```python
from build123d import *

# Parameters (mm, degrees)
F1_DEPTH = 3.175
F2_R     = 3.7719
F3_DEPTH = 1.27
F4_W     = 1.5875
F4_H     = 2.54
F5_DEPTH = 3.175


with BuildPart() as f1:
    # F0 (on Front) → F1 (new body)
    with BuildSketch(Plane.XZ):
        with BuildLine():
            ThreePointArc((39.878, 0), (0, 39.878), (-39.878, 0))
            Line((-39.878, 0), (-39.878, -14.986))
            Line((-39.878, -14.986), (39.878, -14.986))
            Line((39.878, -14.986), (39.878, 0))
        make_face()
    extrude(amount=F1_DEPTH)

    # F2 (on face) → F3 (cut)
    with BuildSketch(Plane.XZ.offset(3.175)):
        with Locations((-12.7, -7.493)):
            Circle(F2_R)
        with Locations((12.7, -7.493)):
            Circle(F2_R)
    extrude(amount=-F3_DEPTH, mode=Mode.SUBTRACT)

    # F4 (on face) → F5 (join)
    with BuildSketch(Plane.XZ.offset(3.175)):
        with Locations((-4.15925, -16.256)):
            Rectangle(F4_W, F4_H)
        with Locations((4.15925, -16.256)):
            Rectangle(F4_W, F4_H)
    extrude(amount=-F5_DEPTH)


solid = f1.part
```
Input: part model. Units: mm. Frame: model coordinates. A direction names the side the tool comes from. Coordinates: 2 decimals unless noted, no trailing zeros. Write each loop counter-clockwise with the first axis right and the second up, starting at its lowest first coordinate (ties: lowest second). Pieces come first, ordered by that corner, then holes.
1) Section B-B on x = -12.7. Output: boundary loops of the cut face in (y, z) (3 decimals), and give its area (3 significant figures).
2) Pin query (flat end, axial travel): pin 1 Ø7 at (x, z) = (12.7, -7.493) entering from +Y; pin 2 Ø2.5 at (x, z) = (12.5, -6.5) entering from -Y (3 decimals); pin 3 Ø0.8 at (y, z) = (-1.5, -16.5) entering from +X; pin 4 Ø0.8 at (y, z) = (-2, -16.5) entering from -X. Return the tip coordinate at first contact, or that it passes through.
3) Section A-A on y = -0.55. Output: boundary loops of the cut face in (x, z).
4) Section D-D on x = 0. Output: boundary loops of the cut face in (y, z) (3 decimals), and give its area (3 significant figures).
5) Mould query, pull axis X, two halves, no side actions, for faces 4 (the cylindrical face through (11.882, -2.549, -11.175)), 5 (the flat face through (4, -2, -17.526)), 6 (the cylindrical face through (0.88, -1.57, 39.87)), 7 (the flat face through (-13, -1.905, -7)). Classes: pulls with the +X half, pulls with the -X half, needs draft (parallel to the pull), parting line crosses it, or undercut.
6) Set-up query: faces 1 (the flat face through (-4.953, -2, -16)), 2 (the flat face through (4.953, -2, -16)), 3 (the flat face through (-3.366, -2, -16)). Return all of +Z, -Z, +X, -X, +Y, -Y with unobstructed straight access to the full face (end or side cutting, diameter ignored); none if empty.
7) Section C-C on z = 14.5. Output: boundary loops of the cut face in (x, y) (3 decimals).
8) Material intervals for line 1 along X through (y, z) = (-2.5, -9); line 2 along Z through (x, y) = (12.7, -2.5); line 3 along Z through (x, y) = (-9.5, -2.4), sorted ascending.
Check result:
1. outline: (-3.175, -14.986) - (0, -14.986) - (0, 37.802) - (-3.175, 37.802) - (-3.175, -3.721) - (-1.905, -3.721) - (-1.905, -11.265) - (-3.175, -11.265) - close
1. area: 158 mm2
2. pin 1: stops at y = 0
2. pin 2: stops at y = -1.905
2. pin 3: stops at x = 4.95
2. pin 4: stops at x = -4.95
3. outline: (-39.88, -14.99) - (-4.95, -14.99) - (-4.95, -17.53) - (-3.37, -17.53) - (-3.37, -14.99) - (3.37, -14.99) - (3.37, -17.53) - (4.95, -17.53) - (4.95, -14.99) - (39.88, -14.99) - (39.88, 0) arc R39.88 ccw to (-39.88, 0) - close
4. outline: (-3.175, -14.986) - (0, -14.986) - (0, 39.878) - (-3.175, 39.878) - close
4. area: 174 mm2
5. face 4: undercut
5. face 5: needs draft
5. face 6: parting line crosses it
5. face 7: undercut
6. face 1: -Z, -X, +Y, -Y
6. face 2: -Z, +X, +Y, -Y
6. face 3: -Z, +Y, -Y
7. outline: (-37.148, -3.175) - (37.148, -3.175) - (37.148, 0) - (-37.148, 0) - close
8. line 1: x = -39.88 to -16.16, -9.24 to 9.24, 16.16 to 39.88
8. line 2: z = -14.99 to -11.26, -3.72 to 37.8
8. line 3: z = -14.99 to -9.49, -5.5 to 38.73
